```python
from build123d import *

# Parameters (mm, degrees)
SKETCH1_W           = 48
SKETCH1_H           = 28
SKETCH1_W_2         = 40
SKETCH1_H_2         = 20
BOSS_EXTRUDE1_DEPTH = 95
SKETCH6_W           = 2.5
SKETCH6_H           = 5
BOSS_EXTRUDE3_DEPTH = 5
SKETCH7_W           = 55.319039298
SKETCH7_H           = 2
CUT_EXTRUDE1_DEPTH  = 20


with BuildPart() as part:
    # Sketch1 → Boss-Extrude1 (new body)
    with BuildSketch(Plane(origin=(0, 0, 0), x_dir=(1, 0, 0), z_dir=(0, 1, 0))):
        with Locations((20, -10)):
            Rectangle(SKETCH1_W, SKETCH1_H)
        with Locations((20, -10)):
            Rectangle(SKETCH1_W_2, SKETCH1_H_2, mode=Mode.SUBTRACT)
    extrude(amount=BOSS_EXTRUDE1_DEPTH)

    # Sketch6 → Boss-Extrude3 (add)
    with BuildSketch(Plane.XZ):
        with Locations((-2.75, 10)):
            Rectangle(SKETCH6_W, SKETCH6_H)
        with Locations((42.75, 10)):
            Rectangle(SKETCH6_W, SKETCH6_H)
    extrude(amount=BOSS_EXTRUDE3_DEPTH)

    # Sketch7 → Cut-Extrude1 (cut)
    with BuildSketch(Plane.XY.offset(24)):
        with Locations((21.062221668, 90)):
            Rectangle(SKETCH7_W, SKETCH7_H)
    extrude(amount=-CUT_EXTRUDE1_DEPTH, mode=Mode.SUBTRACT)


solid = part.part
```
Part model, mm, in its own coordinate system. A direction names the side the tool comes from. Give positions to 0.01 mm unless a question says otherwise; leave off trailing zeros. Order: outer loops, then holes, each group sorted by start corner. A loop starts at its lowest first (then second) coordinate and runs counter-clockwise, first axis right, second up. Notation, with made-up numbers: M 59.5,24.25 L 63.5,24.25 A20 ccw 63.5,39.25 Z; hole C 79.25,73 d5. An arc over 180 degrees is marked long. Use a Markdown table: item, result. Add a question column.
(1) Saw through at A-A, the plane z = 18.5. Give the cut face in (x, y).
(2) Saw through at B-B, the plane x = 10.5. Give the cut face in (y, z).
(3) Drop flat-ended pins along their axis: P1, Ø2, axis at x = -2.5, y = -2.5, coming from the -Z side; P2, Ø1.5, axis at x = 10, z = 19.5, coming from the -Y side; P3, Ø2, axis at x = 42, y = -3, coming from the +Z side. Give the stop position or say it passes through.
(4) Saw through at C-C, the plane y = 57.5. Give the cut face in (x, z), and give its area (3 significant figures).
(5) Probe line 1 along X through (y, z) = (57.5, 1.5); line 2 along Z through (x, y) = (14, 33); line 3 along Y through (x, z) = (36, 20.75). List the from-to ranges inside material, lowest first. Write a range as [from, to].
(6) Mould opens along Y. For faces 1 (the face through (-2, 90, 4)), 2 (the face through (43, -2, 12.5)), 3 (the face through (20, 95, 22)) say: +Y half, -Y half, draft (parallel to the pull), parting line (faces both ways), or undercut.
(7) 3-axis set-ups, long thin cutter, end or side, ignore diameter. For faces 4 (the face through (20, 91, 21)), 5 (the face through (-1.5, -2, 10)), 6 (the face through (20, 47, 0)): which of +Z, -Z, +X, -X, +Y, -Y reach the whole face in a straight line?
Answer key:
| question | item | result |
|---|---|---|
| 1 | outline | M -4,0 L 0,0 L 0,89 L -4,89 Z; M -4,91 L 0,91 L 0,95 L -4,95 Z; M 40,0 L 44,0 L 44,89 L 40,89 Z; M 40,91 L 44,91 L 44,95 L 40,95 Z |
| 2 | outline | M 0,-4 L 95,-4 L 95,0 L 0,0 Z; M 0,20 L 89,20 L 89,24 L 0,24 Z; M 91,20 L 95,20 L 95,24 L 91,24 Z |
| 3 | P1 | z = 7.5 |
| 3 | P2 | y = 0 |
| 3 | P3 | z = 12.5 |
| 4 | outline | M -4,-4 L 44,-4 L 44,24 L -4,24 Z; hole M 0,0 L 40,0 L 40,20 L 0,20 Z |
| 4 | area | 544 mm^2 |
| 5 | line 1 | [-4, 0], [40, 44] |
| 5 | line 2 | [-4, 0], [20, 24] |
| 5 | line 3 | [0, 89], [91, 95] |
| 6 | face 1 | undercut |
| 6 | face 2 | draft |
| 6 | face 3 | +Y half |
| 7 | face 4 | +Z, +X, -X |
| 7 | face 5 | +Z, -Z, -Y |
| 7 | face 6 | +Y, -Y |
